Read the model definition and answer for the solid it produces. Units are mm, in the model's axes. A direction names the side the tool comes from. Give positions to 0.01 mm unless a question says otherwise; leave off trailing zeros. Loops run counter-clockwise (first coordinate to the right, second up) from the corner with the lowest first, then second, coordinate; pieces in that order, holes last. Notation, with made-up numbers: (55, 81.5) - (94, 81.5) arc R23 ccw to (94, 111.5) - close; hole circle Ø7 at (-3, 89.25). An arc over 180 degrees is marked (long way). Use a Markdown table: item, result. Add a question column.
Item 1: For a pull along Z with two mould halves and no side action, classify faces 6 (the face through (0, 4, 2)), 7 (the face through (1.14, 3.51, 5.1)), 8 (the face through (0, 3.5, 3)) as +Z half, -Z half, draft (parallel to the pull), parting line (faces both ways), or undercut.
Item 2: Consider probe 1 along Z at (x, y) = (1.5, 0.55); probe 2 along Y at (x, z) = (1.5, 3.75); probe 3 along X at (y, z) = (3.5, 1.9). Determine where each line is inside the solid, lowest interval first. Write a range as [from, to].
Item 3: A cutting plane is placed at B-B (y = 1.65). Determine the outline of the cut face in (x, z), plus the area to 3 significant figures.
Item 4: A cutting plane is placed at C-C (z = 4.8). Determine the outline of the cut face in (x, y).
Item 5: Which of the six approach directions +Z, -Z, +X, -X, +Y, -Y give full straight-line access (tool end or side, diameter ignored) to faces 1 (the face through (-2, 0, 0.5)), 2 (the face through (1, 0, 0.5)), 3 (the face through (-2, 2, 0)), 4 (the face through (1, 3, 3)), 5 (the face through (-1, 3.5, 1.5))?
Item 6: A cutting plane is placed at D-D (x = -3.5). Determine the outline of the cut face in (y, z), plus the area to 3 significant figures.
Item 7: A cutting plane is placed at A-A (x = -0.75). Determine the outline of the cut face in (y, z), plus the area to 3 significant figures.
Item 8: Each of these flat-tipped pins is pushed along its axis until it touches: P1, Ø0.9, axis at x = 1, z = 4, coming from the -Y side; P2, Ø3, axis at x = -2.5, z = 1.5, coming from the -Y side; P3, Ø0.5, axis at x = 0.5, z = 0.5, coming from the -Y side; P4, Ø0.8, axis at y = 3.5, z = 5, coming from the -X side. Where does it stop, or does it pass through?
from build123d import *

# Parameters (mm, degrees)
BOSS_EXTRUDE1_DEPTH = 1
BOSS_EXTRUDE2_DEPTH = 1


with BuildPart() as part:
    # Sketch1 → Boss-Extrude1 (new body)
    with BuildSketch(Plane.XY):
        with BuildLine():
            Line((0, 0), (2, 0))
            Line((2, 0), (2, 4))
            Line((2, 4), (-4, 4))
            ThreePointArc((-4, 4), (-4.707106781, 3.707106781), (-5, 3))
            Line((-5, 3), (-5, 1))
            Line((-5, 1), (-3, -1))
            Line((-3, -1), (-2, -1))
            Line((-2, -1), (-2, 1))
            ThreePointArc((-2, 1), (-1, 2), (0, 1))
            Line((0, 1), (0, 0))
        make_face()
    extrude(amount=BOSS_EXTRUDE1_DEPTH)

    # Sketch2 → Boss-Extrude2 (add)
    with BuildSketch(Plane(origin=(0, 4, 0), x_dir=(1, 0, 0), z_dir=(0, 1, 0))):
        with BuildLine():
            Line((-1, -1), (2, -1))
            Line((2, -1), (2, -3))
            ThreePointArc((2, -3), (1.121320344, -5.121320344), (-1, -6))
            Line((-1, -6), (-1, -4))
            ThreePointArc((-1, -4), (0, -3), (-1, -2))
            Line((-1, -2), (-1, -1))
        make_face()
    extrude(amount=-BOSS_EXTRUDE2_DEPTH)


solid = part.part
Geometry says:
| question | item | result |
|---|---|---|
| 1 | face 6 | draft |
| 1 | face 7 | +Z half |
| 1 | face 8 | undercut |
| 2 | probe 1 | [0, 1] |
| 2 | probe 2 | [3, 4] |
| 2 | probe 3 | [-1, 2] |
| 3 | outline | (-5, 0) - (-1.76, 0) - (-1.76, 1) - (-5, 1) - close; (-0.24, 0) - (2, 0) - (2, 1) - (-0.24, 1) - close |
| 3 | area | 5.48 mm² |
| 4 | outline | (-1, 3) - (1.4, 3) - (1.4, 4) - (-1, 4) - close |
| 5 | face 1 | +Z, -Z, -Y |
| 5 | face 2 | +Z, -Z, +X, -Y |
| 5 | face 3 | -Z, +X, -X, +Y, -Y |
| 5 | face 4 | +Z, +X, -X, -Y |
| 5 | face 5 | +Z, -X, +Y, -Y |
| 6 | outline | (-0.5, 0) - (4, 0) - (4, 1) - (-0.5, 1) - close |
| 6 | area | 4.50 mm² |
| 7 | outline | (1.97, 0) - (4, 0) - (4, 2.03) - (3, 2.03) - (3, 1) - (1.97, 1) - close; (3, 3.97) - (4, 3.97) - (4, 5.99) - (3, 5.99) - close |
| 7 | area | 5.08 mm² |
| 8 | P1 | y = 3 |
| 8 | P2 | y = -1 |
| 8 | P3 | y = 0 |
| 8 | P4 | x = -1 |
